For this review, take the finished solid that the model builds, in its own axes (mm). A direction names the side the tool comes from. Coordinates: 2 decimals unless noted, no trailing zeros. Loops run counter-clockwise (first coordinate to the right, second up) from the corner with the lowest first, then second, coordinate; pieces in that order, holes last. Notation, with made-up numbers: M 24,63.5 L 79,63.5 A14 ccw 79,76.5 Z; hole C -37,-8 d4. An arc over 180 degrees is marked long. Put each result on its own line as item: value.
Autodesk Fusion 360 part; units mm, degrees
sketch "Skizze1" plane through (0, 0, 0) normal (0, 0, 1) x (1, 0, 0)
  line L0 (0.0185, 31.9947) -> (0.0278, 32)
  line L1 (-1.9679, 35.4635) -> (-7.7548, 45.5067)
  line L2 (-29.6959, 19.4899) -> (-35.4814, 29.5308)
  line L3 (-43.2796, 25.0376) -> (-27.6989, 16.024)
  line L4 (-0.7462, 33.3433) -> (0.0278, 32)
  line L5 (0.0278, 32) -> (0.8041, 33.3419)
  line L6 (0.0093, 16) -> (-27.6989, 16.024)
  line L7 (-7.7548, 45.5067) -> (-22.7322, 71.5005)
  line L8 (-35.4814, 29.5308) -> (-50.4589, 55.5246)
  line L9 (-22.7322, 71.5005) -> (-50.4589, 55.5246)
  line L10 (-22.7322, 71.5005) -> (-14.9341, 75.9937)
  line L11 (-43.2796, 25.0376) -> (-58.257, 51.0313)
  line L12 (-50.4589, 55.5246) -> (-58.257, 51.0313)
  line L13 (0.0434, 74.9415) -> (0, 0)
  line L14 (35.5156, 29.4897) -> (50.5231, 55.4661)
  line L15 (22.815, 71.4741) -> (15.022, 75.9764)
  line L16 (0.0093, 16) -> (27.7175, 15.992)
  line L17 (7.8074, 45.4977) -> (22.815, 71.4741)
  line L18 (29.7185, 19.4555) -> (35.5156, 29.4897)
  line L19 (43.3085, 24.9874) -> (27.7175, 15.992)
  line L20 (50.5231, 55.4661) -> (58.3161, 50.9638)
  line L21 (22.815, 71.4741) -> (50.5231, 55.4661)
  line L22 (43.3085, 24.9874) -> (58.3161, 50.9638)
  line L23 (2.0103, 35.4635) -> (7.8074, 45.4977)
  line L24 (15.022, 75.9764) -> (-14.9341, 75.9937)
  line L25 (29.7185, 19.4555) -> (2.0103, 35.4635)
  line L26 (-29.6959, 19.4899) -> (-29.2073, 19.4555)
  line L27 (-29.2073, 19.4555) -> (-1.9679, 35.4635)
  line L28 (0.0185, 31.9947) -> (0.0093, 32)
  line L29 (0.0434, 50) -> (0.029, 50.025)
  line L30 (0.0145, 50) -> (0.029, 50.025)
  line L31 (-29.2073, 19.4555) -> (-29.5555, 19.2509)
  line L32 (-29.6959, 19.4899) -> (-29.5555, 19.2509)
  dimension "d1" = 50
  dimension "d2" = 32
  dimension "d8" = 30
  dimension "d10" = 30
extrude "Extrusion3" add sketch "Skizze1" along normal blind 4 contours L1 L2 L3 L6 L7 L8 L10 L11 L12 L14 L15 L16 L17 L18 L19 L20 L22 L23 L24 L25 L27 L31 L32
extrude "Extrusion4" add sketch "Skizze1" along normal blind 3 contours L1 L2 L7 L8 L9 L26 L27 | L14 L17 L18 L21 L23 L25
extrude "Extrusion5" add 1 faces at (0.6994, 62.4779, 4) along direction (0, 0, 1) blind 3
hole "Bohrung1" at (0.0504, 56.8999, 7) direction (0, 0, -1) diameter 6 depth 8 tip angle 118
sketch "Skizze2" plane through (0, 0, 7) normal (0, 0, 1) x (-1, 0, 0)
  circle A0 centre (-0.0504, -56.8999) radius 3
  line L0 (-0.0278, -32) -> (-0.0185, -31.9947)
  line L1 (-0.0185, -31.9947) -> (-0.0185, -32.016)
  line L2 (-0.0185, -32.016) -> (-0.0278, -32)
  line L3 (29.6959, -19.4899) -> (50.4589, -55.5246)
  line L4 (50.4589, -55.5246) -> (58.257, -51.0313)
  line L5 (58.257, -51.0313) -> (43.2796, -25.0376)
  line L6 (43.2796, -25.0376) -> (27.6989, -16.024)
  line L7 (27.6989, -16.024) -> (-0.0093, -16)
  line L8 (-0.0093, -16) -> (-27.7175, -15.992)
  line L9 (-27.7175, -15.992) -> (-43.3085, -24.9874)
  line L10 (-43.3085, -24.9874) -> (-58.3161, -50.9638)
  line L11 (-58.3161, -50.9638) -> (-50.5231, -55.4661)
  line L12 (-50.5231, -55.4661) -> (-29.7185, -19.4555)
  line L13 (-29.7185, -19.4555) -> (-2.0103, -35.4635)
  line L14 (-2.0103, -35.4635) -> (-22.815, -71.4741)
  line L15 (-22.815, -71.4741) -> (-15.022, -75.9764)
  line L16 (-15.022, -75.9764) -> (14.9341, -75.9937)
  line L17 (14.9341, -75.9937) -> (22.7322, -71.5005)
  line L18 (22.7322, -71.5005) -> (1.9679, -35.4635)
  line L19 (1.9679, -35.4635) -> (29.5555, -19.2509)
  line L20 (29.5555, -19.2509) -> (29.6959, -19.4899)
  line L21 (-15.8644, -15.9954) -> (-0.4521, -24.8996)
  line L22 (13.8448, -16.012) -> (-0.4521, -24.8996)
extrude "Extrusion6" cut sketch "Skizze2" against normal blind 23 contours L7 L8 L21 L22
sketch "Skizze3" plane through (0, 0, 3) normal (0, 0, 1) x (-1, 0, 0)
  line L0 (29.6959, -19.4899) -> (29.2073, -19.4555)
  line L1 (29.2073, -19.4555) -> (1.9679, -35.4635)
  line L2 (1.9679, -35.4635) -> (22.7322, -71.5005)
  line L3 (22.7322, -71.5005) -> (50.4589, -55.5246)
  line L4 (50.4589, -55.5246) -> (29.6959, -19.4899)
  line L5 (18.7813, -25.5826) -> (13.6085, -28.6226)
  line L6 (18.7813, -25.5826) -> (13.1225, -15.9535)
  line L7 (13.6085, -28.6226) -> (7.9138, -18.9326)
  line L8 (7.9138, -18.9326) -> (13.1225, -15.9535)
  line L9 (-0.0434, -74.9415) -> (0, 0)
  line L10 (-13.6416, -28.6068) -> (-7.9358, -18.9234)
  line L11 (-7.9358, -18.9234) -> (-13.1409, -15.9383)
  line L12 (-18.8109, -25.5609) -> (-13.1409, -15.9383)
  line L13 (-18.8109, -25.5609) -> (-13.6416, -28.6068)
  dimension "d23" = 6
  dimension "d24" = 12.5
extrude "Extrusion7" cut sketch "Skizze3" along normal mid plane 26 contours L1 L5 L6 L7 L8 | L10 L11 L12 L13
extrude "Extrusion8" cut 1 faces at (17.0878, 26.5762, 2.3333) along direction (0.507661, 0.861557, 0) blind 0.5
(1) For pin 1 (3 mm diameter, centred on y = 27, z = 5, fed in from +X); pin 2 (3 mm diameter, centred on x = 4, z = 5, fed in from +Y); pin 3 (4 mm diameter, centred on y = 32, z = 6, fed in from +X), all flat-tipped, find the tip position at first contact; note any pin that passes through.
Determined:
pin 1: stops at x = 45.34
pin 2: stops at y = 75.98
pin 3: stops at x = 48.52
(2) Tool access review of faces 1 (the flat face through (-27, 46, 3)), 2 (the flat face through (35.62, 20.55, 3.45)), 3 (the flat face through (-3.957, 22.159, 3.549)), 4 (the flat face through (-16.2, 27.1, 1.5)): name each direction out of +Z, -Z, +X, -X, +Y, -Y from which nothing blocks a thin tool from reaching the whole face with its end or side.
Determined:
face 1: +Z
face 2: +Z, -Z, +X, -Y
face 3: +Z, -Z, -Y
face 4: +Z, -Z
(3) Add section C-C (y = 42). Write out the cut boundary in (x, z), plus the area to 3 significant figures.
Determined:
outline: M -53.05,0 L 53.14,0 L 53.14,7 L 42.74,7 L 42.74,3 L 5.79,3 L 5.79,7 L -5.73,7 L -5.73,3 L -42.67,3 L -42.67,7 L -53.05,7 Z
area: 448 mm^2
(4) Wall thickness on line 1 along X through (y, z) = (23, 6.5); line 2 along X through (y, z) = (54.5, 5.75); line 3 along Z through (x, y) = (33.5, 37.5): over which ranges is each line inside the solid? List them lowest first. Write a range as [from, to].
Determined:
line 1: x = [-39.76, -31.72], [-23.18, -17.26], [-10.3, -2.6], [3.74, 10.34], [17.3, 23.58], [31.77, 39.86]
line 2: x = [-52.24, -49.87], [-12.94, -1.75], [1.85, 13.01], [49.96, 52.2]
line 3: z = [0, 3]
(5) Draft analysis for pull direction Y (two halves, no side actions). For faces 5 (the flat face through (26, 46, 3)), 6 (the flat face through (-41, 33, 7)), 7 (the flat face through (4.615, 22.495, 3.549)), state which applies: +Y half, -Y half, draft (parallel to the pull), parting line (faces both ways), or undercut.
Determined:
face 5: undercut
face 6: draft
face 7: -Y half
(6) Add section A-A (y = 61). Write out the cut boundary in (x, z).
Determined:
outline: M -40.96,0 L 40.94,0 L 40.94,3 L 16.76,3 L 16.76,7 L -16.68,7 L -16.68,3 L -40.96,3 Z
